Source: CAD feature listing. Evaluate the final solid. Frame: model axes, mm. A direction names the side the tool comes from. Coordinates: 2 decimals unless noted, no trailing zeros. Write each loop counter-clockwise with the first axis right and the second up, starting at its lowest first coordinate (ties: lowest second). Pieces come first, ordered by that corner, then holes. Notation, with made-up numbers: (-2.5, -22.5) -> (42.5, -22.5) arc R25 cw to (42.5, 9.5) -> close; hole circle Ø10 at (28, -36.75). An arc over 180 degrees is marked (long way). Write item = value, one per line.
from build123d import *

# Parameters (mm, degrees)
BASESTEELANGLE_DEPTH        = 12.7
F_1_4_CLEARANCE_HOLE1_D     = 6.7564
F_1_4_CLEARANCE_SLOT1_DEPTH = 3.175


# Read off the part's stored shape, not the designer's step: 1/4 Clearance Slot1
with BuildPart() as part:
    # Sketch1 → BaseSteelAngle (new, symmetric)
    with BuildSketch(Plane.XY):
        with BuildLine():
            Line((0, 0), (0, 38.1))
            Line((0, 38.1), (0.00508, 38.1))
            ThreePointArc((0.00508, 38.1), (2.246551928, 37.171551928), (3.175, 34.93008))
            Line((3.175, 34.93008), (3.175, 7.9375))
            ThreePointArc((3.175, 7.9375), (4.569903955, 4.569903955), (7.9375, 3.175))
            Line((7.9375, 3.175), (34.93008, 3.175))
            ThreePointArc((34.93008, 3.175), (37.171551928, 2.246551928), (38.1, 0.00508))
            Line((38.1, 0.00508), (38.1, 0))
            Line((38.1, 0), (0, 0))
        make_face()
    extrude(amount=BASESTEELANGLE_DEPTH, both=True)

    # 1/4 Clearance Hole1 (through all)
    with Locations(Plane(origin=(25.40508, 3.175, 0), x_dir=(1, 0, 0), z_dir=(0, 1, 0))):
        with Locations((0, 0)):
            Hole(F_1_4_CLEARANCE_HOLE1_D / 2)

    # 1/4 Clearance Slot1 outline → 1/4 Clearance Slot1 (cut)
    with BuildSketch(Plane.YZ):
        with BuildLine():
            Line((24.40559, 3.3782), (18.46199, 3.3782))
            ThreePointArc((18.46199, 3.3782), (15.08379, 0), (18.46199, -3.3782))
            Line((18.46199, -3.3782), (24.40559, -3.3782))
            ThreePointArc((24.40559, -3.3782), (27.78379, 0), (24.40559, 3.3782))
        make_face()
    extrude(amount=F_1_4_CLEARANCE_SLOT1_DEPTH, mode=Mode.SUBTRACT)


solid = part.part
1) Cut plane C-C, the plane x = 23. Output: boundary loops of the cut face in (y, z) (3 decimals), and give its area (3 significant figures).
Answer block:
outline = (0, -12.7) -> (3.175, -12.7) -> (3.175, -2.372) -> (0, -2.372) -> close; (0, 2.372) -> (3.175, 2.372) -> (3.175, 12.7) -> (0, 12.7) -> close
area = 65.6 mm2
2) First-contact query: pin 1 Ø3 at (y, z) = (5.5, 5) entering from +X; pin 2 Ø2 at (x, z) = (20.5, -5.5) entering from +Y (3 decimals); pin 3 Ø4 at (x, z) = (25.41, 0) entering from -Y; pin 4 Ø8 at (y, z) = (4.5, 1.5) entering from +X. Flat tips, straight axial feed; report the tip coordinate or a pass-through.
Answer block:
pin_1 = 5.26
pin_2 = 3.175
pin_3 = through
pin_4 = 38.06
3) Cut plane B-B, the plane z = 0. Give the number of separate pieces and of enclosed holes in the cut face, and give its area (3 significant figures).
Answer block:
separate_pieces = 3
enclosed_holes = 0
area = 171 mm2
4) Pull-direction query (Y, two-part tool) for faces 4 (the flat face through (21, 3.175, 0)), 5 (the cylindrical face through (1.565, 15.085, 0.074)), 6 (the flat face through (11, 2, -12.7)), 7 (the cylindrical face through (1.565, 27.783, -0.074)); classes: +Y half, -Y half, draft (parallel to the pull), parting line (faces both ways), or undercut.
Answer block:
face_4 = +Y half
face_5 = undercut
face_6 = draft
face_7 = undercut
5) Cut plane A-A, the plane y = 19. Output: boundary loops of the cut face in (x, z) (3 decimals), and give its area (3 significant figures).
Answer block:
outline = (0, -12.7) -> (3.175, -12.7) -> (3.175, -3.378) -> (0, -3.378) -> close; (0, 3.378) -> (3.175, 3.378) -> (3.175, 12.7) -> (0, 12.7) -> close
area = 59.2 mm2
6) Material intervals for probe 1 along Y at (x, z) = (35, 2.5); probe 2 along X at (y, z) = (24.5, 4.25) (3 decimals); probe 3 along Y at (x, z) = (37, 10.25), sorted ascending. Write a range as [from, to].
Answer block:
probe_1 = [0, 3.17]
probe_2 = [0, 3.175]
probe_3 = [0, 2.41]
7) Reachability of faces 1 (the flat face through (19, 0, 0)), 2 (the flat face through (2, 21, 3.378)), 3 (the flat face through (3.175, 22, -5)) from +Z, -Z, +X, -X, +Y, -Y: full face, straight path, thin tool, end or side. Return the list, or none.
Answer block:
face_1 = +Z, -Z, +X, -X, -Y
face_2 = +X, -X
face_3 = +Z, -Z, +X, +Y
